```python
from build123d import *

# Parameters (mm, degrees)
SKETCH1_W            = 40
SKETCH1_H            = 36
BOSS_EXTRUDE1_DEPTH  = 2.81
M4_CLEARANCE_HOLE1_D = 4.5
M6_CLEARANCE_HOLE1_D = 6.6


with BuildPart() as part:
    # Sketch1 → Boss-Extrude1 (new body)
    with BuildSketch(Plane.XY):
        Rectangle(SKETCH1_W, SKETCH1_H)
    extrude(amount=BOSS_EXTRUDE1_DEPTH)

    # M4 Clearance Hole1 (through all)
    with Locations(Plane(origin=(0, 0, 0), x_dir=(-1, 0, 0), z_dir=(0, 0, -1))):
        with Locations((-15.273020567, -10.999999997), (-15.273020567, 11.110907406)):
            Hole(M4_CLEARANCE_HOLE1_D / 2)

    # M6 Clearance Hole1 (through all)
    with Locations(Plane(origin=(0, 0, 0), x_dir=(-1, 0, 0), z_dir=(0, 0, -1))):
        with Locations((5.877074643, -10.111576322), (5.877074643, 11.282650508)):
            Hole(M6_CLEARANCE_HOLE1_D / 2)


solid = part.part
```
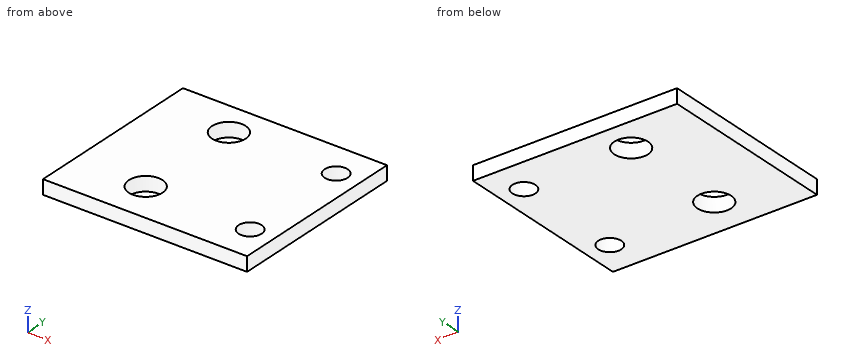
The listing builds one solid part. Answer for the finished solid, in the listing's coordinates (mm). Round coordinates to 2 decimals unless told otherwise and drop trailing zeros. Loops run counter-clockwise (first coordinate to the right, second up) from the corner with the lowest first, then second, coordinate; pieces in that order, holes last.
1) Given P1, Ø2.5, axis at x = 15.27, y = -11, coming from the -Z side, flat-ended and moving along its own axis, determine where the tip first touches the part or whether it passes through.
Outcome:
P1: passes through
2) A cutting plane is placed at B-B on z = 0.6. Determine the outline of the cut face in (x, y), plus the area to 3 significant figures.
Outcome:
outline: (-20, -18) - (20, -18) - (20, 18) - (-20, 18) - close; hole circle Ø6.6 at (-5.88, -10.11); hole circle Ø6.6 at (-5.88, 11.28); hole circle Ø4.5 at (15.27, -11); hole circle Ø4.5 at (15.27, 11.11)
area: 1,340 mm2
3) Consider line 1 (Y direction, x = 17, z = 0.6); line 2 (Y direction, x = -6, z = 0.2); line 3 (X direction, y = -9.5, z = 0.9). Determine where each line is inside the solid, lowest interval first.
Outcome:
line 1: y = -18 to -12.44, -9.56 to 9.67, 12.55 to 18
line 2: y = -18 to -13.41, -6.81 to 7.98, 14.58 to 18
line 3: x = -20 to -9.12, -2.63 to 13.6, 16.95 to 20
4) A cutting plane is placed at A-A on y = -11. Determine the outline of the cut face in (x, z).
Outcome:
outline: (-20, 0) - (-9.06, 0) - (-9.06, 2.81) - (-20, 2.81) - close; (-2.7, 0) - (13.02, 0) - (13.02, 2.81) - (-2.7, 2.81) - close; (17.52, 0) - (20, 0) - (20, 2.81) - (17.52, 2.81) - close
